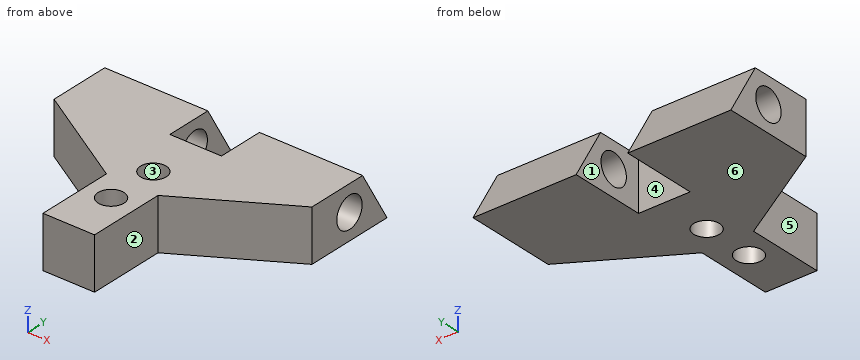
from build123d import *

# Parameters (mm, degrees)
ESQUISSE1_R             = 2.5
BOSS_EXTRU_1_DEPTH      = 10
ENL_V_MAT_EXTRU_1_REACH = 61.034
ESQUISSE2_R             = 3


with BuildPart() as part:
    # Esquisse1 → Boss.-Extru.1 (new body)
    with BuildSketch(Plane.XY):
        Polygon((-25, 12), (-5, 0), (-5, -15), (5, -15), (5, 0), (25, 12), (25, 29.75), (5, 29.75), (5, 15), (-5, 15), (-5, 29.75), (-25, 29.75), align=None)
        with Locations((0, -5)):
            Circle(ESQUISSE1_R, mode=Mode.SUBTRACT)
        with Locations((0, 5)):
            Circle(ESQUISSE1_R, mode=Mode.SUBTRACT)
    extrude(amount=BOSS_EXTRU_1_DEPTH)

    # Enlèv. mat.-Extru.1: up to this face of the body (flat: up to its plane)
    enl_v_mat_extru_1_end = Plane(part.part.faces().sort_by_distance((25, 20.875, 5))[0])
    # Esquisse2 → Enlèv. mat.-Extru.1 (cut, up to the picked face)
    with BuildSketch(Plane.ZY.offset(25), mode=Mode.PRIVATE) as enl_v_mat_extru_1_sk1:
        with Locations((5, 20.875)):
            Circle(ESQUISSE2_R)
    enl_v_mat_extru_1_tool1 = split(extrude(enl_v_mat_extru_1_sk1.sketch, amount=-ENL_V_MAT_EXTRU_1_REACH, mode=Mode.PRIVATE), bisect_by=enl_v_mat_extru_1_end, keep=Keep.BOTH, mode=Mode.PRIVATE)
    # Esquisse2 → Enlèv. mat.-Extru.1 (cut, up to the picked face)
    with BuildSketch(Plane.ZY.offset(25), mode=Mode.PRIVATE) as enl_v_mat_extru_1_sk2:
        Polygon((0, 29.75), (10, 29.75), (10, 23.976497308), align=None)
    enl_v_mat_extru_1_tool2 = split(extrude(enl_v_mat_extru_1_sk2.sketch, amount=-ENL_V_MAT_EXTRU_1_REACH, mode=Mode.PRIVATE), bisect_by=enl_v_mat_extru_1_end, keep=Keep.BOTH, mode=Mode.PRIVATE)
    add(enl_v_mat_extru_1_tool1.solids().sort_by(Axis((-25, 20.875, 5), (1, 0, 0)))[0], mode=Mode.SUBTRACT)
    add(enl_v_mat_extru_1_tool2.solids().sort_by(Axis((-25, 27.825499, 6.666667), (1, 0, 0)))[0], mode=Mode.SUBTRACT)


solid = part.part
Geometry: final body of the model. Coordinates: model frame, mm. Face numbers are marked on the shaded views. A direction names the side the tool comes from. Give positions to 0.01 mm unless a question says otherwise; leave off trailing zeros. Loops run counter-clockwise (first coordinate to the right, second up) from the corner with the lowest first, then second, coordinate; pieces in that order, holes last. Notation, with made-up numbers: (68.5, -18.5) - (106.5, -18.5) arc R7 cw to (106.5, -7.5) - close; hole circle Ø1 at (-25, 84.5). An arc over 180 degrees is marked (long way). One line per question, with ' | ' between items. Start each with the question number.
(1) Ray query, line 1 (Y direction, x = 0, z = 7); line 2 (X direction, y = 4, z = 8); line 3 (Z direction, x = -16.5, y = 22.5). Return the intervals inside material, ascending. Write a range as from..to.
(2) Reachability of the marked faces 1, 2 and 3 from +Z, -Z, +X, -X, +Y, -Y: full face, straight path, thin tool, end or side. Return the list, or none.
(3) Section query C-C on z = 3. Return loops of the section in (x, y), then the cut area to 3 significant figures.
(4) Section query B-B on x = 0. Return loops of the section in (y, z).
(5) Contact query for flat-ended pins moving along their axis: pin 1 (3.5 mm diameter, centred on y = 20.875, z = 5, fed in from -X); pin 2 (4 mm diameter, centred on x = 7.5, z = 4.5, fed in from +Y); pin 3 (3 mm diameter, centred on y = -6.5, z = 7.5, fed in from +X); pin 4 (3 mm diameter, centred on x = -1, z = 4, fed in from +Y). Output: stop coordinate, or through.
(6) Section query D-D on z = 9.25. Return loops of the section in (x, y).
(7) Pull-direction query (X, two-part tool) for the marked faces 4, 5 and 6; classes: released by +X, released by -X, zero draft, split by the parting line, or undercut.
(8) Section query A-A on y = -5. Return loops of the section in (x, z), then the cut area to 3 significant figures.
The answers:
1) line 1: -15..-7.5, -2.5..2.5, 7.5..15 | line 2: -11.67..-2.29, 2.29..11.67 | line 3: 0..2.48, 7.52..10
2) face 1: +Z, -Z, +Y | face 2: +Z, -Z, +X, -Y | face 3: +Z, -Z
3) outline: (-25, 12) - (-5, 0) - (-5, -15) - (5, -15) - (5, 0) - (25, 12) - (25, 18.64) - (5, 18.64) - (5, 15) - (-5, 15) - (-5, 18.64) - (-25, 18.64) - close; (-25, 23.11) - (-5, 23.11) - (-5, 28.02) - (-25, 28.02) - close; (5, 23.11) - (25, 23.11) - (25, 28.02) - (5, 28.02) - close; hole circle Ø5 at (0, -5); hole circle Ø5 at (0, 5) | area: 963 mm2
4) outline: (-15, 0) - (-7.5, 0) - (-7.5, 10) - (-15, 10) - close; (-2.5, 0) - (2.5, 0) - (2.5, 10) - (-2.5, 10) - close; (7.5, 0) - (15, 0) - (15, 10) - (7.5, 10) - close
5) pin 1: through | pin 2: y = 28.31 | pin 3: x = 5 | pin 4: y = 15
6) outline: (-25, 12) - (-5, 0) - (-5, -15) - (5, -15) - (5, 0) - (25, 12) - (25, 24.41) - (5, 24.41) - (5, 15) - (-5, 15) - (-5, 24.41) - (-25, 24.41) - close; hole circle Ø5 at (0, -5); hole circle Ø5 at (0, 5)
7) face 4: undercut | face 5: released by -X | face 6: zero draft
8) outline: (-5, 0) - (-2.5, 0) - (-2.5, 10) - (-5, 10) - close; (2.5, 0) - (5, 0) - (5, 10) - (2.5, 10) - close | area: 50.0 mm2
